from build123d import *

# Parameters (mm, degrees)
SKETCH2_R           = 100
SKETCH2_R_2         = 4.25
BOSS_EXTRUDE1_DEPTH = 58
SKETCH3_R           = 7
CUT_EXTRUDE1_DEPTH  = 8
CUT_EXTRUDE2_START  = -28
CUT_EXTRUDE2_DEPTH  = 28
BOSS_EXTRUDE2_DEPTH = 50


with BuildPart() as part:
    # Sketch2 → Boss-Extrude1 (new body)
    with BuildSketch(Plane(origin=(0, 0, 0), x_dir=(1, 0, 0), z_dir=(0, 1, 0))):
        with Locations(Location((0, 0, 0), (0, 0, 90))):
            Circle(SKETCH2_R)
        with Locations(Location((0, 84.5, 0), (0, 0, 90))):
            Circle(SKETCH2_R_2, mode=Mode.SUBTRACT)
        with Locations(Location((84.5, 0, 0), (0, 0, 90))):
            Circle(SKETCH2_R_2, mode=Mode.SUBTRACT)
        with Locations(Location((0, -84.5, 0), (0, 0, 90))):
            Circle(SKETCH2_R_2, mode=Mode.SUBTRACT)
        with Locations(Location((-84.5, 0, 0), (0, 0, 90))):
            Circle(SKETCH2_R_2, mode=Mode.SUBTRACT)
    extrude(amount=BOSS_EXTRUDE1_DEPTH)

    # Sketch3 → Cut-Extrude1 (cut)
    with BuildSketch(Plane(origin=(0, 58, 0), x_dir=(1, 0, 0), z_dir=(0, 1, 0))):
        with Locations(Location((0, 84.5, 0), (0, 0, 270))):
            Circle(SKETCH3_R)
        with Locations(Location((84.5, 0, 0), (0, 0, 270))):
            Circle(SKETCH3_R)
        with Locations(Location((0, -84.5, 0), (0, 0, 270))):
            Circle(SKETCH3_R)
        with Locations(Location((-84.5, 0, 0), (0, 0, 270))):
            Circle(SKETCH3_R)
    extrude(amount=-CUT_EXTRUDE1_DEPTH, mode=Mode.SUBTRACT)

    # Sketch4 → Cut-Extrude2 (cut)
    with BuildSketch(Plane(origin=(0, 58, 0), x_dir=(1, 0, 0), z_dir=(0, 1, 0)).offset(CUT_EXTRUDE2_START)):
        with BuildLine():
            Line((-25, 68.053287944), (-25, 96.824583655))
            ThreePointArc((-25, 96.824583655), (-70.710678119, 70.710678119), (-96.824583655, 25))
            Line((-96.824583655, 25), (-68.053287944, 25))
            ThreePointArc((-68.053287944, 25), (-51.265241636, 51.265241636), (-25, 68.053287944))
        make_face()
        with BuildLine():
            Line((68.053287944, 25), (96.824583655, 25))
            ThreePointArc((96.824583655, 25), (70.710678119, 70.710678119), (25, 96.824583655))
            Line((25, 96.824583655), (25, 68.053287944))
            ThreePointArc((25, 68.053287944), (51.265241636, 51.265241636), (68.053287944, 25))
        make_face()
        with BuildLine():
            ThreePointArc((25, -96.824583655), (70.710678119, -70.710678119), (96.824583655, -25))
            Line((96.824583655, -25), (68.053287944, -25))
            ThreePointArc((68.053287944, -25), (51.265241636, -51.265241636), (25, -68.053287944))
            Line((25, -68.053287944), (25, -96.824583655))
        make_face()
        with BuildLine():
            ThreePointArc((-96.824583655, -25), (-70.710678119, -70.710678119), (-25, -96.824583655))
            Line((-25, -96.824583655), (-25, -68.053287944))
            ThreePointArc((-25, -68.053287944), (-51.265241636, -51.265241636), (-68.053287944, -25))
            Line((-68.053287944, -25), (-68.372754715, -25))
            Line((-68.372754715, -25), (-96.824583655, -25))
        make_face()
    extrude(amount=CUT_EXTRUDE2_DEPTH, mode=Mode.SUBTRACT)

    # Sketch5 → Boss-Extrude2 (add)
    with BuildSketch(Plane(origin=(0, 58, 0), x_dir=(1, 0, 0), z_dir=(0, 1, 0))):
        with BuildLine():
            Line((-36.538461538, 6.319875664), (-13.461538462, 21.066252212))
            ThreePointArc((-13.461538462, 21.066252212), (0, 22.912467498), (13.461538462, 21.066252212))
            Line((13.461538462, 21.066252212), (36.538461538, 6.319875664))
            ThreePointArc((36.538461538, 6.319875664), (40, 0), (36.538461538, -6.319875664))
            Line((36.538461538, -6.319875664), (13.461538462, -21.066252212))
            ThreePointArc((13.461538462, -21.066252212), (0, -22.912467498), (-13.461538462, -21.066252212))
            Line((-13.461538462, -21.066252212), (-36.538461538, -6.319875664))
            ThreePointArc((-36.538461538, -6.319875664), (-40, 0), (-36.538461538, 6.319875664))
        make_face()
    extrude(amount=BOSS_EXTRUDE2_DEPTH)


solid = part.part
The model under review builds one solid part; all positions refer to its coordinate system, in mm. A direction names the side the tool comes from. Give positions to 0.01 mm unless a question says otherwise; leave off trailing zeros. Write each loop counter-clockwise with the first axis right and the second up, starting at its lowest first coordinate (ties: lowest second). Pieces come first, ordered by that corner, then holes.
1. Add section A-A, the plane x = 0. Write out the cut boundary in (y, z), plus the area to 3 significant figures.
2. Draft analysis for pull direction Z (two halves, no side actions). For faces 6 (the cylindrical face through (91.44, 54.06, -0.91)), 7 (the cylindrical face through (0.308, 54.056, -91.493)), 8 (the flat face through (-61, 30, 60)), 9 (the cylindrical face through (51.58, 43.8, 50.95)), state which applies: +Z half, -Z half, draft (parallel to the pull), parting line (faces both ways), or undercut.
3. Add section C-C, the plane y = 10. Write out the cut boundary in (x, z), plus the area to 3 significant figures.
4. Tool access review of faces 1 (the cylindrical face through (-40, 83, 0)), 2 (the flat face through (83, 44, 25)), 3 (the flat face through (-83, 44, -25)), 4 (the cylindrical face through (40, 83, 0)), 5 (the cylindrical face through (-50.95, 43.8, 51.58)): name each direction out of +Z, -Z, +X, -X, +Y, -Y from which nothing blocks a thin tool from reaching the whole face with its end or side.
5. Add section B-B, the plane z = 0. Write out the cut boundary in (x, y), plus the area to 3 significant figures.
6. Add section D-D, the plane z = -84.5. Write out the cut boundary in (x, y), plus the area to 3 significant figures.
7. Wall thickness on L1, parallel to X at y = 55, z = 0; L2, parallel to Z at x = 84.5, y = 34; L3, parallel to X at y = 56, z = -84.5: over which ranges is each line inside the solid? List them lowest first.
8. For P1, Ø16, axis at x = -84.5, z = 0, coming from the +Y side; P2, Ø6, axis at y = 25.5, z = 40.5, coming from the -X side; P3, Ø4, axis at x = 77.5, y = 14, coming from the +Z side, all flat-tipped, find the tip position at first contact; note any pin that passes through.
Worked answers:
1. outline: (0, -100) - (58, -100) - (58, -91.5) - (50, -91.5) - (50, -88.75) - (0, -88.75) - close; (0, -80.25) - (50, -80.25) - (50, -77.5) - (58, -77.5) - (58, -22.91) - (108, -22.91) - (108, 22.91) - (58, 22.91) - (58, 77.5) - (50, 77.5) - (50, 80.25) - (0, 80.25) - close; (0, 88.75) - (50, 88.75) - (50, 91.5) - (58, 91.5) - (58, 100) - (0, 100) - close
1. area: 12,800 mm2
2. face 6: undercut
2. face 7: undercut
2. face 8: draft
2. face 9: +Z half
3. outline: circle Ø200 at (0, 0); hole circle Ø8.5 at (-84.5, 0); hole circle Ø8.5 at (0, -84.5); hole circle Ø8.5 at (0, 84.5); hole circle Ø8.5 at (84.5, 0)
3. area: 31,200 mm2
4. face 1: -X, +Y
4. face 2: +Z, +X, +Y
4. face 3: -Z, -X, +Y
4. face 4: +X, +Y
4. face 5: +Z, -X, +Y
5. outline: (-100, 0) - (-88.75, 0) - (-88.75, 50) - (-91.5, 50) - (-91.5, 58) - (-100, 58) - close; (-80.25, 0) - (80.25, 0) - (80.25, 50) - (77.5, 50) - (77.5, 58) - (40, 58) - (40, 108) - (-40, 108) - (-40, 58) - (-77.5, 58) - (-77.5, 50) - (-80.25, 50) - close; (88.75, 0) - (100, 0) - (100, 58) - (91.5, 58) - (91.5, 50) - (88.75, 50) - close
5. area: 14,500 mm2
6. outline: (-53.48, 0) - (-4.25, 0) - (-4.25, 50) - (-7, 50) - (-7, 58) - (-25, 58) - (-25, 30) - (-53.48, 30) - close; (4.25, 0) - (53.48, 0) - (53.48, 30) - (25, 30) - (25, 58) - (7, 58) - (7, 50) - (4.25, 50) - close
6. area: 4,070 mm2
7. L1: x = -100 to -91.5, -77.5 to 77.5, 91.5 to 100
7. L2: z = -25 to -4.25, 4.25 to 25
7. L3: x = -25 to -7, 7 to 25
8. P1: stops at y = 58
8. P2: stops at x = -92.7
8. P3: stops at z = 65.57
